Could you check a few things on this model? Use its own coordinates, in mm. Face numbers are marked on the shaded views. A direction names the side the tool comes from. Give positions to 0.01 mm unless a question says otherwise; leave off trailing zeros.
(1) Will these pins go through, and if not, where does the flat tip stop? pin 1 (3 mm diameter, centred on y = 29, z = -54, fed in from +X); pin 2 (4 mm diameter, centred on x = 1.5, z = -2.5, fed in from -Y); pin 3 (8 mm diameter, centred on x = -105, z = 130.5, fed in from -Y).
(2) On a 3-axis mill with a long thin cutter (end or side, diameter ignored), from which of +Z, -Z, +X, -X, +Y, -Y can I reach the whole of each face in a straight line? I mean the marked faces 1 and 2. Say none if no direction works.
(3) If I drill on probe 1 along X at (y, z) = (88, 0) (1 decimal); probe 2 along X at (y, z) = (96, -12); probe 3 along Y at (x, z) = (-66, -192), over which ranges is the centre line in solid material (lowest first)?
(4) Imagine slicing it at A-A, the plane y = 89. State how many separate pieces and enclosed holes the cut face has, then the cut area to 3 significant figures.
from build123d import *

# Parameters (mm, degrees)
BOSS_EXTRUDE1_REACH      = 319.128
BOSS_EXTRUDE1_END_RADIUS = 348.751469298
SKETCH2_R                = 28.575
CUT_EXTRUDE1_REACH       = 319.128
CUT_EXTRUDE1_END_RADIUS  = 348.751469298
SKETCH3_R                = 20.955
SKETCH3_R_2              = 19.3675
CUT_EXTRUDE2_REACH       = 319.128
CUT_EXTRUDE2_END_RADIUS  = 348.751469298
SKETCH6_R                = 6.985
BOSS_EXTRUDE4_DEPTH      = 19.05
SKETCH7_R                = 5.715
CUT_EXTRUDE3_DEPTH       = 16.51


with BuildPart() as part:
    # Sketch1 → Revolve1 (revolve)
    with BuildSketch(Plane.XY):
        with BuildLine():
            Line((212.725, 0), (191.135, 0))
            ThreePointArc((191.135, 0), (99.243909749, 39.232491681), (0, 50.8))
            Line((0, 50.8), (0, 72.39))
            ThreePointArc((0, 72.39), (112.352389522, 53.796868331), (212.725, 0))
        make_face()
    revolve(axis=Axis((0, 0, 0), (0, -1, 0)))

    # Boss-Extrude1: up to this sphere (the profile starts outside it)
    boss_extrude1_end = Location((0, -276.361469298, 0)) * Sphere(BOSS_EXTRUDE1_END_RADIUS, mode=Mode.PRIVATE)
    # Sketch2 → Boss-Extrude1 (add, up to the surface)
    with BuildSketch(Plane(origin=(0, 100.33, 0), x_dir=(1, 0, 0), z_dir=(0, 1, 0)), mode=Mode.PRIVATE) as boss_extrude1_sk1:
        with Locations(Location((0, 0, 0), (0, 0, 270))):
            Circle(SKETCH2_R)
    boss_extrude1_tool1 = extrude(boss_extrude1_sk1.sketch, amount=-BOSS_EXTRUDE1_REACH, mode=Mode.PRIVATE) - boss_extrude1_end
    add(boss_extrude1_tool1.solids().sort_by_distance((0, 100.33, 0))[0])

    # Cut-Extrude1: up to this sphere (the profile starts outside it)
    cut_extrude1_end = Location((0, -276.361469298, 0)) * Sphere(CUT_EXTRUDE1_END_RADIUS, mode=Mode.PRIVATE)
    # Sketch3 → Cut-Extrude1 (cut, up to the surface)
    with BuildSketch(Plane(origin=(0, 100.33, 0), x_dir=(1, 0, 0), z_dir=(0, 1, 0)), mode=Mode.PRIVATE) as cut_extrude1_sk1:
        with Locations(Location((0, 0, 0), (0, 0, 270))):
            Circle(SKETCH3_R)
        with Locations(Location((0, 0, 0), (0, 0, 270))):
            Circle(SKETCH3_R_2, mode=Mode.SUBTRACT)
    cut_extrude1_tool1 = extrude(cut_extrude1_sk1.sketch, amount=-CUT_EXTRUDE1_REACH, mode=Mode.PRIVATE) - cut_extrude1_end
    add(cut_extrude1_tool1.solids().sort_by_distance((0, 100.33, -20.362303))[0], mode=Mode.SUBTRACT)

    # Cut-Extrude2: up to this sphere (the profile starts outside it)
    cut_extrude2_end = Location((0, -276.361469298, 0)) * Sphere(CUT_EXTRUDE2_END_RADIUS, mode=Mode.PRIVATE)
    # Sketch4 → Cut-Extrude2 (cut, up to the surface)
    with BuildSketch(Plane(origin=(0, 100.33, 0), x_dir=(1, 0, 0), z_dir=(0, 1, 0)), mode=Mode.PRIVATE) as cut_extrude2_sk1:
        with BuildLine():
            Line((-19.302328875, 1.5875), (0, 1.5875))
            Line((0, 1.5875), (0, -1.5875))
            Line((0, -1.5875), (-19.302328875, -1.5875))
            ThreePointArc((-19.302328875, -1.5875), (-19.959892905, 0), (-19.302328875, 1.5875))
        make_face()
    cut_extrude2_tool1 = extrude(cut_extrude2_sk1.sketch, amount=-CUT_EXTRUDE2_REACH, mode=Mode.PRIVATE) - cut_extrude2_end
    add(cut_extrude2_tool1.solids().sort_by_distance((-9.878619, 100.33, 0))[0], mode=Mode.SUBTRACT)

    # Sketch6 → Boss-Extrude4 (add)
    with BuildSketch(Plane(origin=(0, 51.308, 0), x_dir=(1, 0, 0), z_dir=(0, 1, 0))):
        with Locations(Location((0, 0, 0), (0, 0, 270))):
            Circle(SKETCH6_R)
    extrude(amount=-BOSS_EXTRUDE4_DEPTH)

    # Sketch7 → Cut-Extrude3 (cut)
    with BuildSketch(Plane.XZ.offset(-32.258)):
        with Locations(Location((0, 0, 0), (0, 0, 270))):
            Circle(SKETCH7_R)
    extrude(amount=-CUT_EXTRUDE3_DEPTH, mode=Mode.SUBTRACT)


solid = part.part
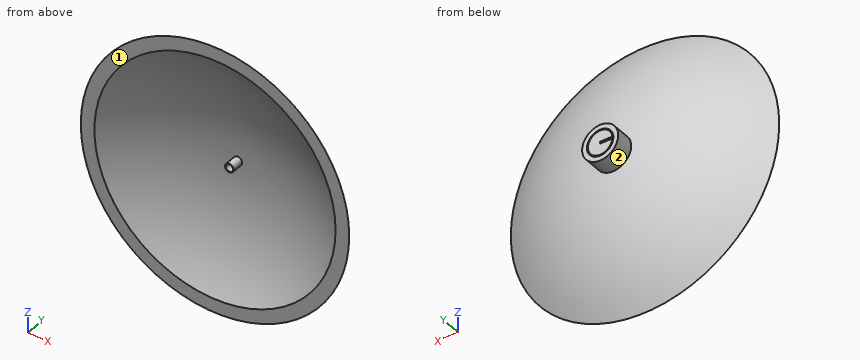
Answer block:
1. pin 1: stops at x = 162.46
1. pin 2: stops at y = 48.77
1. pin 3: stops at y = 11.11
2. face 1: +Z, -Z, +X, -X, -Y
2. face 2: +Y
3. probe 1: x = -28.6 to -21, 0 to 19.4, 21 to 28.6
3. probe 2: x = -25.93 to -17.18, -15.2 to 15.2, 17.18 to 25.93
3. probe 3: y = 0 to 7.2
4. separate pieces: 2
4. enclosed holes: 1
4. area: 2,300 mm2
